Build history of the part. All positions in model axes, mm. Face numbers are marked on the shaded views. A direction names the side the tool comes from. Give positions to 0.01 mm unless a question says otherwise; leave off trailing zeros. Write each loop counter-clockwise with the first axis right and the second up, starting at its lowest first coordinate (ties: lowest second). Pieces come first, ordered by that corner, then holes. Notation, with made-up numbers: (72.5, 26.25) -> (101.5, 26.25) arc R22 ccw to (101.5, 56.25) -> close; hole circle Ø2 at (57, 51.25). An arc over 180 degrees is marked (long way). Put each result on its own line as item: value.
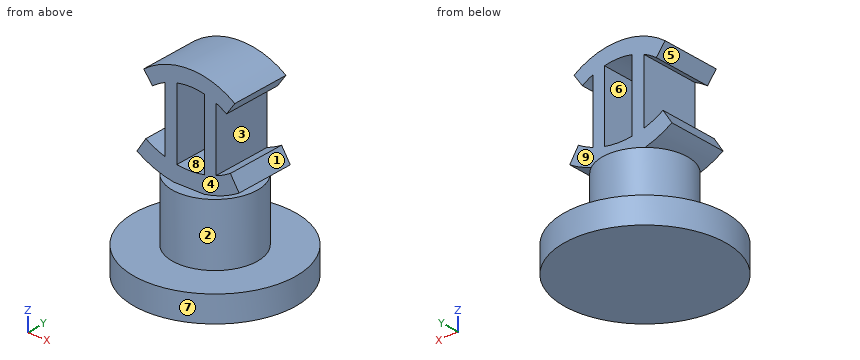
from build123d import *

# Parameters (mm, degrees)
F0_W     = 32.1691036224
F0_H     = 10.3981345892
F2_R     = 16.9245679208
F3_DEPTH = 35.052
F5_DEPTH = 12.446
F6_DEPTH = 11.684


with BuildPart() as f1:
    # F0 (on Front) → F1 (revolve)
    with BuildSketch(Plane.XZ):
        with Locations((16.0845518112, 5.1990672946)):
            Rectangle(F0_W, F0_H)
    revolve(axis=Axis((0, 0, 5.1990672946), (0, 0, -1)))

    # F2 (on Top) → F3 (join)
    with BuildSketch(Plane.XY):
        Circle(F2_R)
    extrude(amount=F3_DEPTH)

    # F4 (on Front) → F5 (join)
    with BuildSketch(Plane.XZ):
        with BuildLine():
            Line((-17.2026802681, 46.2241524707), (-20.7758424342, 40.6702971151))
            ThreePointArc((-20.7758424342, 40.6702971151), (-0.2905255832, 34.5539512873), (20.2953913573, 40.3226527435))
            Line((20.2953913573, 40.3226527435), (16.8152843817, 45.9352860484))
            ThreePointArc((16.8152843817, 45.9352860484), (-0.2354935112, 41.1577205632), (-17.2026802681, 46.2241524707))
        make_face()
        with BuildLine():
            ThreePointArc((-9.4536782582, 42.6405122732), (-13.4477491949, 44.1737830783), (-17.2026802681, 46.2241524707))
            ThreePointArc((-17.2026802681, 46.2241524707), (-0.2354935112, 41.1577205632), (16.8152843817, 45.9352860484))
            ThreePointArc((16.8152843817, 45.9352860484), (13.9600425927, 44.3798005754), (10.962201674, 43.1208762102))
            ThreePointArc((10.962201674, 43.1208762102), (8.6813208555, 42.3910598969), (6.3524134113, 41.833171668))
            ThreePointArc((6.3524134113, 41.833171668), (0.8301071261, 41.2162515517), (-4.7159024645, 41.5601043652))
            ThreePointArc((-4.7159024645, 41.5601043652), (-7.1052467262, 42.0106036166), (-9.4536782582, 42.6405122732))
        make_face()
        with BuildLine():
            Line((-9.4536782582, 68.3503676295), (-9.4536782582, 42.6405122732))
            ThreePointArc((-9.4536782582, 42.6405122732), (-7.1052467262, 42.0106036166), (-4.7159024645, 41.5601043652))
            Line((-4.7159024645, 41.5601043652), (-4.7159024645, 69.8749349594))
            ThreePointArc((-4.7159024645, 69.8749349594), (-7.1217660809, 69.2275577769), (-9.4536782582, 68.3503676295))
        make_face()
        with BuildLine():
            ThreePointArc((6.3524134113, 41.833171668), (8.6813208555, 42.3910598969), (10.962201674, 43.1208762102))
            Line((10.962201674, 43.1208762102), (10.962201674, 68.3503676295))
            ThreePointArc((10.962201674, 68.3503676295), (8.6926434954, 69.2074051813), (6.3524134113, 69.8467257929))
            Line((6.3524134113, 69.8467257929), (6.3524134113, 41.833171668))
        make_face()
        with BuildLine():
            ThreePointArc((-14.4961847769, 65.4524759376), (-12.0571318242, 67.0444552804), (-9.4536782582, 68.3503676295))
            ThreePointArc((-9.4536782582, 68.3503676295), (-7.1217660809, 69.2275577769), (-4.7159024645, 69.8749349594))
            ThreePointArc((-4.7159024645, 69.8749349594), (0.8197914056, 70.4634778759), (6.3524134113, 69.8467257929))
            ThreePointArc((6.3524134113, 69.8467257929), (8.6926434954, 69.2074051813), (10.962201674, 68.3503676295))
            ThreePointArc((10.962201674, 68.3503676295), (13.155285497, 67.2753192406), (15.2364689754, 65.9970309232))
            ThreePointArc((15.2364689754, 65.9970309232), (0.2813076758, 70.5751050434), (-14.4961847769, 65.4524759376))
        make_face()
        with BuildLine():
            Line((-18.0290771655, 70.1051802942), (-14.4961847769, 65.4524759376))
            ThreePointArc((-14.4961847769, 65.4524759376), (0.2813076758, 70.5751050434), (15.2364689754, 65.9970309232))
            Line((15.2364689754, 65.9970309232), (18.5930212877, 70.7785100912))
            ThreePointArc((18.5930212877, 70.7785100912), (0.1721303263, 76.4160867046), (-18.0290771655, 70.1051802942))
        make_face()
    extrude(amount=F5_DEPTH)

    # F6 (add): a face of the model
    f6_faces = [f1.faces().sort_by_distance(p)[0] for p in [
        (-13.6924417201, 0, 43.6446778209),
    ]]
    extrude(f6_faces, amount=F6_DEPTH)


solid = f1.part
1) Slice it at B-B (x = 10). Write the cut outline in (y, z), plus the area to 3 significant figures.
Filled sheet:
outline: (-30.58, 0) -> (30.58, 0) -> (30.58, 10.4) -> (13.65, 10.4) -> (13.65, 35.05) -> (-13.65, 35.05) -> (-13.65, 10.4) -> (-30.58, 10.4) -> close; (-12.45, 35.87) -> (11.68, 35.87) -> (11.68, 75.01) -> (-12.45, 75.01) -> close
area: 2,250 mm2
2) Slice it at D-D (x = -11). Write the cut outline in (y, z), plus the area to 3 significant figures.
Filled sheet:
outline: (-30.23, 0) -> (30.23, 0) -> (30.23, 10.4) -> (12.86, 10.4) -> (12.86, 35.05) -> (-12.86, 35.05) -> (-12.86, 10.4) -> (-30.23, 10.4) -> close; (-12.45, 36.17) -> (11.68, 36.17) -> (11.68, 43.16) -> (-12.45, 43.16) -> close; (-12.45, 67.62) -> (11.68, 67.62) -> (11.68, 74.12) -> (-12.45, 74.12) -> close
area: 1,590 mm2
3) Pull direction X, two halves, no side cores. Call the marked faces 6, 7, 8 and 9: released by +X, released by -X, zero draft, split by the parting line, or undercut.
Filled sheet:
face 6: undercut
face 7: split by the parting line
face 8: undercut
face 9: zero draft
4) Slice it at C-C (y = 0). Write the cut outline in (x, z), plus the area to 3 significant figures.
Filled sheet:
outline: (-32.17, 0) -> (32.17, 0) -> (32.17, 10.4) -> (16.92, 10.4) -> (16.92, 35.05) -> (6.21, 35.05) arc R38.46 ccw to (20.3, 40.32) -> (16.82, 45.94) arc R32.13 cw to (10.96, 43.12) -> (10.96, 68.35) arc R25.71 cw to (15.24, 66) -> (18.59, 70.78) arc R31.05 ccw to (-18.03, 70.11) -> (-14.5, 65.45) arc R25.71 cw to (-9.45, 68.35) -> (-9.45, 42.64) arc R32.13 cw to (-17.2, 46.22) -> (-20.78, 40.67) arc R38.46 ccw to (-6.14, 35.05) -> (-16.92, 35.05) -> (-16.92, 10.4) -> (-32.17, 10.4) -> close; hole (-4.72, 41.56) arc R32.13 ccw to (6.35, 41.83) -> (6.35, 69.85) arc R25.71 ccw to (-4.72, 69.87) -> close
area: 2,220 mm2
5) Slice it at A-A (z = 48.5). Write the cut outline in (x, y), plus the area to 3 significant figures.
Filled sheet:
outline: (-9.45, -12.45) -> (-4.72, -12.45) -> (-4.72, 11.68) -> (-9.45, 11.68) -> close; (6.35, -12.45) -> (10.96, -12.45) -> (10.96, 11.68) -> (6.35, 11.68) -> close
area: 226 mm2
6) Pin check, flat tips, straight feed: pin 1 (5 mm diameter, centred on y = 5, z = 25.5, fed in from -X); pin 2 (1.5 mm diameter, centred on y = 9.5, z = 24, fed in from -X); pin 3 (12 mm diameter, centred on y = -13.5, z = 43, fed in from -X); pin 4 (8 mm diameter, centred on y = 16, z = 51.5, fed in from +X). Stop position of each tip, or through.
Filled sheet:
pin 1: x = -16.74
pin 2: x = -14.49
pin 3: x = -20.78
pin 4: through
7) Wall check: L1, parallel to X at y = -9, z = 46; L2, parallel to X at y = -7, z = 60; L3, parallel to Z at x = 18, y = -13.5. Give the ranges that are in metal, low to high.
Filled sheet:
L1: -17.35 to -16.85, -9.45 to -4.72, 6.35 to 10.96
L2: -9.45 to -4.72, 6.35 to 10.96
L3: 0 to 10.4
8) Tool access for the marked faces 1, 2, 3, 4 and 5: list every direction of +Z, -Z, +X, -X, +Y, -Y with a clear straight run to the whole face (end or side of a thin tool).
Filled sheet:
face 1: +X, +Y, -Y
face 2: none
face 3: +Y, -Y
face 4: +Z, +X, -X, -Y
face 5: -X, +Y, -Y
